Could you check a few things on this drawing? It's one solid part, dimensions in mm from its lowest x, y, z. A direction names the side the tool comes from. Give positions to 0.01 mm unless a question says otherwise; leave off trailing zeros. Write each loop counter-clockwise with the first axis right and the second up, starting at its lowest first coordinate (ties: lowest second). Pieces come first, ordered by that corner, then holes.
1. Suppose I cut it at A-A (x = 2). Please give me the cut outline in (y, z), and give its area (3 significant figures).
2. If I drill on probe 1 along X at (y, z) = (1.4, 7); probe 2 along Z at (x, y) = (18.1, 10.65); probe 3 along X at (y, z) = (10.5, 8.75), over which ranges is the centre line in solid material (lowest first)?
3. Suppose I cut it at D-D (x = 34). Please give me the cut outline in (y, z), and give its area (3 significant figures).
4. I'm going to push flat-ended pins straight in: pin 1 (6.5 mm diameter, centred on x = 14, y = 4.5, fed in from -Z); pin 2 (2 mm diameter, centred on x = 11, z = 2.5, fed in from -Y); pin 3 (8 mm diameter, centred on x = 9.5, z = 5.5, fed in from +Y); pin 4 (3 mm diameter, centred on x = 41.6, z = 7, fed in from +Y). Where does each tip first touch, or does it pass through?
5. Thinking about a two-plate mould opening in X: for the marked faces 5, 6 and 7, which applies, pulls with the +X half, pulls with the -X half, needs draft (parallel to the pull), parting line crosses it, or undercut?
6. On a 3-axis mill with a long thin cutter (end or side, diameter ignored), from which of +Z, -Z, +X, -X, +Y, -Y can I reach the whole of each face in a straight line? I mean the marked faces 1, 2, 3 and 4. Say none if no direction works.
7. Suppose I cut it at C-C (y = 1.5). Please give me the cut outline in (x, z).
8. Suppose I cut it at B-B (z = 8.75). Please give me the cut outline in (x, y), and give its area (3 significant figures).
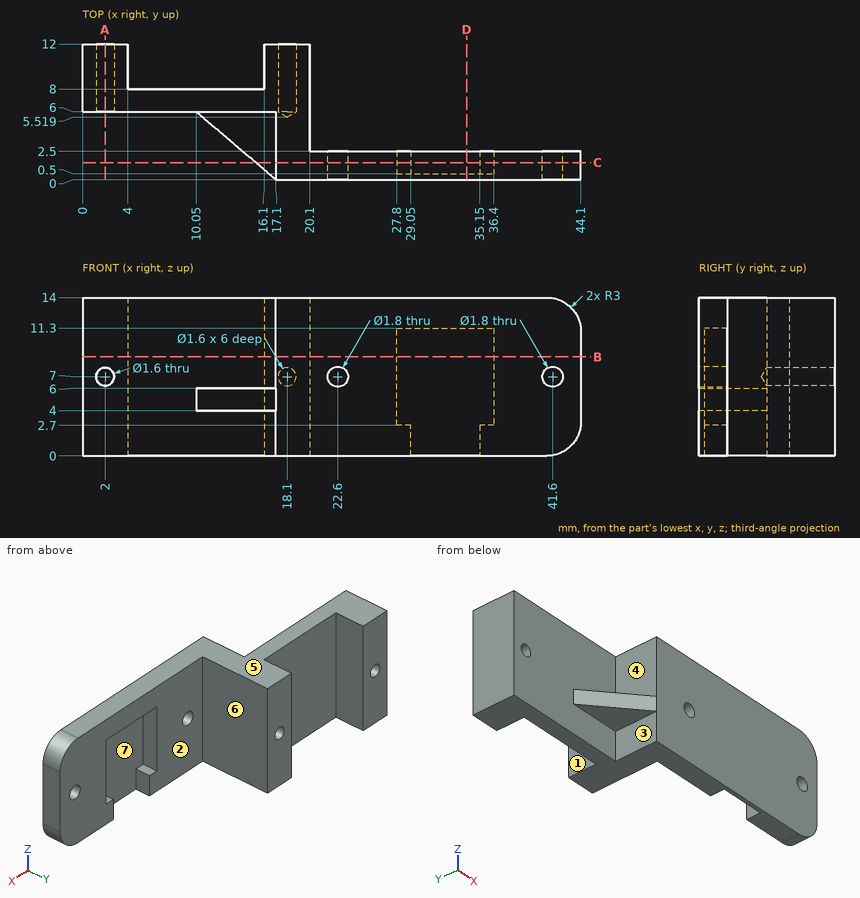
Checks:
1. outline: (6, 0) - (12, 0) - (12, 6.2) - (6, 6.2) - close; (6, 7.8) - (12, 7.8) - (12, 14) - (6, 14) - close
1. area: 74.4 mm2
2. probe 1: x = 17.1 to 21.7, 23.5 to 27.8, 36.4 to 40.7, 42.5 to 44.1
2. probe 2: z = 0 to 6.2, 7.8 to 14
2. probe 3: x = 0 to 4, 16.1 to 20.1
3. outline: (0, 0) - (0.5, 0) - (0.5, 11.3) - (2.5, 11.3) - (2.5, 14) - (0, 14) - close
3. area: 12.4 mm2
4. pin 1: stops at z = 0
4. pin 2: stops at y = 6
4. pin 3: stops at y = 8
4. pin 4: stops at y = 2.5
5. face 5: needs draft
5. face 6: pulls with the +X half
5. face 7: undercut
6. face 1: +Z, -Z, +Y
6. face 2: +Z, -Z, +X, +Y
6. face 3: -Z, -X, -Y
6. face 4: +Z, -X, -Y
7. outline: (15.34, 4) - (17.1, 4) - (17.1, 0) - (29.05, 0) - (29.05, 2.7) - (27.8, 2.7) - (27.8, 11.3) - (36.4, 11.3) - (36.4, 2.7) - (35.15, 2.7) - (35.15, 0) - (41.1, 0) arc R3 ccw to (44.1, 3) - (44.1, 11) arc R3 ccw to (41.1, 14) - (17.1, 14) - (17.1, 6) - (15.34, 6) - close; hole circle Ø1.8 at (22.6, 7); hole circle Ø1.8 at (41.6, 7)
8. outline: (0, 6) - (17.1, 6) - (17.1, 0) - (44.1, 0) - (44.1, 2.5) - (36.4, 2.5) - (36.4, 0.5) - (27.8, 0.5) - (27.8, 2.5) - (20.1, 2.5) - (20.1, 12) - (16.1, 12) - (16.1, 8) - (4, 8) - (4, 12) - (0, 12) - close
8. area: 133 mm2
